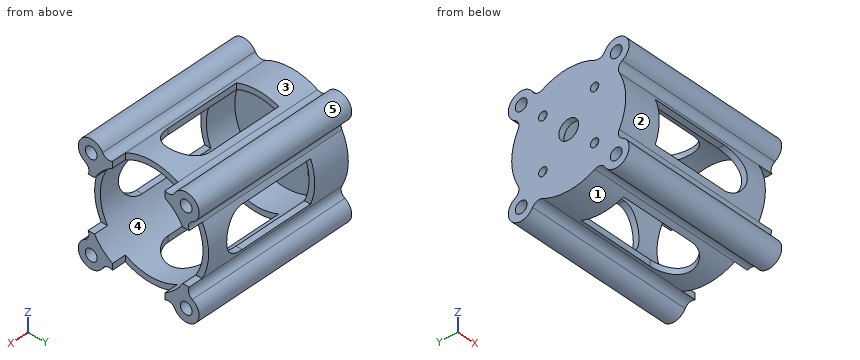
from build123d import *

# Parameters (mm, degrees)
SKETCH_1_R               = 20.25
EXTRUDE_1_DEPTH          = 2
SKETCH_2_R               = 3.5
CUT_EXTRUDE_1_DEPTH      = 3
SKETCH_3_R               = 20.25
SKETCH_3_R_2             = 10.25
EXTRUDE_2_DEPTH          = 4.1
SKETCH_5_R               = 20.25
SKETCH_5_R_2             = 16.25
EXTRUDE_3_DEPTH          = 5.4
SKETCH_6_R               = 20.25
SKETCH_6_R_2             = 18.25
EXTRUDE_4_DEPTH          = 47.5
SKETCH_7_R               = 1.5
CUT_EXTRUDE_2_DEPTH      = 60
PATTERN_CIRCULAR_1_COUNT = 4
FILLET_1_R               = 0.5
SKETCH_9_R               = 4.6
SKETCH_9_R_2             = 2.1
EXTRUDE_6_DEPTH          = 59
EXTRUDE_7_DEPTH          = 59
PATTERN_CIRCULAR_3_COUNT = 4
CUT_EXTRUDE_3_DEPTH      = 22.464496731
PATTERN_CIRCULAR_4_COUNT = 2
PATTERN_CIRCULAR_4_ANGLE = 270
SKETCH_22_R              = 18.25
CUT_EXTRUDE_9_DEPTH      = 20
SKETCH_23_W              = 5
SKETCH_23_H              = 18.640041254
CUT_EXTRUDE_10_DEPTH     = 43.928993463
PATTERN_CIRCULAR_5_COUNT = 2
PATTERN_CIRCULAR_5_ANGLE = 270


with BuildPart() as part:
    # Эскиз1 → Бобышка-Вытянуть1 (new body)
    with BuildSketch(Plane(origin=(0, 0, 0), x_dir=(0, 0, -1), z_dir=(1, 0, 0))):
        Circle(SKETCH_1_R)
    extrude(amount=EXTRUDE_1_DEPTH)

    # Эскиз2 → Вырез-Вытянуть1 (cut, through all)
    with BuildSketch(Plane.ZY):
        Circle(SKETCH_2_R)
    extrude(amount=-CUT_EXTRUDE_1_DEPTH, mode=Mode.SUBTRACT)

    # Эскиз3 → Бобышка-Вытянуть2 (add)
    with BuildSketch(Plane(origin=(2, 0, 0), x_dir=(0, 0, -1), z_dir=(1, 0, 0))):
        Circle(SKETCH_3_R)
        Circle(SKETCH_3_R_2, mode=Mode.SUBTRACT)
    extrude(amount=EXTRUDE_2_DEPTH)

    # Эскиз5 → Бобышка-Вытянуть3 (add)
    with BuildSketch(Plane(origin=(6.1, 0, 0), x_dir=(0, 0, -1), z_dir=(1, 0, 0))):
        Circle(SKETCH_5_R)
        Circle(SKETCH_5_R_2, mode=Mode.SUBTRACT)
    extrude(amount=EXTRUDE_3_DEPTH)

    # Эскиз6 → Бобышка-Вытянуть4 (add)
    with BuildSketch(Plane(origin=(11.5, 0, 0), x_dir=(0, 0, -1), z_dir=(1, 0, 0))):
        Circle(SKETCH_6_R)
        Circle(SKETCH_6_R_2, mode=Mode.SUBTRACT)
    extrude(amount=EXTRUDE_4_DEPTH)

    # Эскиз7 → Вырез-Вытянуть2 (cut, through all)
    with BuildSketch(Plane.ZY):
        with Locations((-9.192388155, 9.192388155)):
            Circle(SKETCH_7_R)
    cut_extrude_2 = extrude(amount=-CUT_EXTRUDE_2_DEPTH, mode=Mode.SUBTRACT)

    # Круговой массив1: Вырез-Вытянуть2 ×4 about axis
    pattern_circular_1_axis = Axis((0, 0, 0), (1, 0, 0))
    for i in range(1, PATTERN_CIRCULAR_1_COUNT):
        add(cut_extrude_2.rotate(pattern_circular_1_axis, i * 360 / PATTERN_CIRCULAR_1_COUNT), mode=Mode.SUBTRACT)

    # Скругление1
    fillet_1_edges = [part.edges().sort_by_distance(p)[0] for p in [
        (2, 0, 10.25),
        (6.1, 0, 10.25),
        (6.1, 0, 16.25),
        (11.5, 0, 16.25),
        (11.5, 0, 18.25),
    ]]
    fillet(fillet_1_edges, radius=FILLET_1_R)

    # Эскиз9 → Бобышка-Вытянуть6 (add)
    with BuildSketch(Plane.ZY):
        with Locations((-16.864496731, 16.864496731)):
            Circle(SKETCH_9_R)
        with Locations((-16.864496731, 16.864496731)):
            Circle(SKETCH_9_R_2, mode=Mode.SUBTRACT)
    extrude_6 = extrude(amount=-EXTRUDE_6_DEPTH)

    # Эскиз10 → Бобышка-Вытянуть7 (add)
    with BuildSketch(Plane.ZY):
        with BuildLine():
            ThreePointArc((-9.320020627, 17.977756131), (-11.289373131, 17.800047957), (-12.818708454, 19.053468456))
            ThreePointArc((-12.818708454, 19.053468456), (-12.323239372, 17.597287013), (-12.335539952, 16.059170405))
            ThreePointArc((-12.335539952, 16.059170405), (-10.870191755, 17.085123096), (-9.320020627, 17.977756131))
        make_face()
        with BuildLine():
            ThreePointArc((-16.059170405, 12.335539952), (-17.597287013, 12.323239372), (-19.053468456, 12.818708454))
            ThreePointArc((-19.053468456, 12.818708454), (-17.800047957, 11.289373131), (-17.977756131, 9.320020627))
            ThreePointArc((-17.977756131, 9.320020627), (-17.085123096, 10.870191755), (-16.059170405, 12.335539952))
        make_face()
    extrude_7 = extrude(amount=-EXTRUDE_7_DEPTH)

    # Круговой массив3: Бобышка-Вытянуть6, Бобышка-Вытянуть7 ×4 about axis
    pattern_circular_3_axis = Axis((0, 0, 0), (1, 0, 0))
    for i in range(1, PATTERN_CIRCULAR_3_COUNT):
        add(extrude_6.rotate(pattern_circular_3_axis, i * 360 / PATTERN_CIRCULAR_3_COUNT))
        add(extrude_7.rotate(pattern_circular_3_axis, i * 360 / PATTERN_CIRCULAR_3_COUNT))

    # Эскиз11 → Вырез-Вытянуть3 (cut, symmetric)
    with BuildSketch(Plane(origin=(0, 0, 0), x_dir=(1, 0, 0), z_dir=(0, 1, 0))):
        with BuildLine():
            Line((13, 7.5), (39.5, 7.5))
            ThreePointArc((39.5, 7.5), (47, 0), (39.5, -7.5))
            Line((39.5, -7.5), (13, -7.5))
            Line((13, -7.5), (13, 7.5))
        make_face()
    cut_extrude_3 = extrude(amount=CUT_EXTRUDE_3_DEPTH, both=True, mode=Mode.SUBTRACT)

    # Круговой массив4: Вырез-Вытянуть3 ×2 about axis
    pattern_circular_4_axis = Axis((2, 0, 0), (-1, 0, 0))
    for i in range(1, PATTERN_CIRCULAR_4_COUNT):
        add(cut_extrude_3.rotate(pattern_circular_4_axis, i * PATTERN_CIRCULAR_4_ANGLE / (PATTERN_CIRCULAR_4_COUNT - 1)), mode=Mode.SUBTRACT)

    # Эскиз22 → Вырез-Вытянуть9 (cut)
    with BuildSketch(Plane(origin=(2, 0, 0), x_dir=(0, 0, -1), z_dir=(1, 0, 0))):
        Circle(SKETCH_22_R)
    extrude(amount=CUT_EXTRUDE_9_DEPTH, mode=Mode.SUBTRACT)

    # Эскиз23 → Вырез-Вытянуть10 (cut, through all)
    with BuildSketch(Plane(origin=(0, -21.464496731, 0), x_dir=(-1, 0, 0), z_dir=(0, -1, 0))):
        with Locations((-56.5, 0)):
            Rectangle(SKETCH_23_W, SKETCH_23_H)
    cut_extrude_10 = extrude(amount=-CUT_EXTRUDE_10_DEPTH, mode=Mode.SUBTRACT)

    # Круговой массив5: Вырез-Вытянуть10 ×2 about axis
    pattern_circular_5_axis = Axis((2, 0, 0), (-1, 0, 0))
    for i in range(1, PATTERN_CIRCULAR_5_COUNT):
        add(cut_extrude_10.rotate(pattern_circular_5_axis, i * PATTERN_CIRCULAR_5_ANGLE / (PATTERN_CIRCULAR_5_COUNT - 1)), mode=Mode.SUBTRACT)


solid = part.part
Input: part model. Units: mm. Frame: model coordinates. Face numbers are marked on the shaded views. A direction names the side the tool comes from. Coordinates: 2 decimals unless noted, no trailing zeros. Loops run counter-clockwise (first coordinate to the right, second up) from the corner with the lowest first, then second, coordinate; pieces in that order, holes last.
(1) Section D-D on x = 10.5. Return the cut outline in (y, z), then the cut area to 3 significant figures.
(2) Section B-B on z = 5.5. Return the cut outline in (x, y), then the cut area to 3 significant figures.
(3) Pull-direction query (Z, two-part tool) for the marked faces 1, 2 and 3; classes: released by +Z, released by -Z, zero draft, split by the parting line, or undercut.
(4) Set-up query: the marked faces 4 and 5. Return all of +Z, -Z, +X, -X, +Y, -Y with unobstructed straight access to the full face (end or side cutting, diameter ignored); none if empty.
(5) Material intervals for probe 1 along Z at (x, y) = (39.5, -18); probe 2 along Y at (x, z) = (19.5, 15); probe 3 along X at (y, z) = (-5, -3), sorted ascending.
(6) Section A-A on y = 0. Return the cut outline in (x, z), then the cut area to 3 significant figures.
(7) First-contact query: pin 1 Ø1.4 at (y, z) = (-1, -18) entering from +X; pin 2 Ø3 at (x, z) = (51.5, 10) entering from -Y; pin 3 Ø1.1 at (x, y) = (22.5, 18) entering from -Z. Flat tips, straight axial feed; report the tip coordinate or a pass-through.
Data:
1. outline: (-19.05, -12.82) arc R4.6 ccw (long way) to (-12.82, -19.05) arc R2.61 cw to (-9.32, -17.98) arc R20.25 ccw to (9.32, -17.98) arc R2.61 cw to (12.82, -19.05) arc R4.6 ccw (long way) to (19.05, -12.82) arc R2.61 cw to (17.98, -9.32) arc R20.25 ccw to (17.98, 9.32) arc R2.61 cw to (19.05, 12.82) arc R4.6 ccw (long way) to (12.82, 19.05) arc R2.61 cw to (9.32, 17.98) arc R20.25 ccw to (-9.32, 17.98) arc R2.61 cw to (-12.82, 19.05) arc R4.6 ccw (long way) to (-19.05, 12.82) arc R2.61 cw to (-17.98, 9.32) arc R20.25 ccw to (-17.98, -9.32) arc R2.61 cw to start; hole circle Ø4.2 at (-16.86, -16.86); hole circle Ø4.2 at (-16.86, 16.86); hole circle Ø36.5 at (0, 0); hole circle Ø4.2 at (16.86, -16.86); hole circle Ø4.2 at (16.86, 16.86)
1. area: 457 mm2
2. outline: (0, -19.49) - (13, -19.49) - (13, -17.4) - (2, -17.4) - (2, 17.4) - (13, 17.4) - (13, 19.49) - (0, 19.49) - close; (44.6, -19.49) - (54, -19.49) - (54, -17.4) - (44.6, -17.4) - close; (44.6, 17.4) - (54, 17.4) - (54, 19.49) - (44.6, 19.49) - close
2. area: 163 mm2
3. face 1: released by -Z
3. face 2: undercut
3. face 3: released by +Z
4. face 4: +X
4. face 5: +X, -X
5. probe 1: z = -21.32 to -18.63, -15.1 to -11.77, -9.28 to -7.5, 7.5 to 9.28, 11.77 to 15.1, 18.63 to 21.32
5. probe 2: y = -21.07 to -17.83, -15.9 to -10.4, 10.4 to 15.9, 17.83 to 21.07
5. probe 3: x = 0 to 2
6. outline: (0, -20.25) - (13, -20.25) - (13, -18.25) - (2, -18.25) - (2, -3.5) - (0, -3.5) - close; (0, 3.5) - (2, 3.5) - (2, 18.25) - (13, 18.25) - (13, 20.25) - (0, 20.25) - close; (47, -20.25) - (54, -20.25) - (54, -18.25) - (47, -18.25) - close; (47, 18.25) - (54, 18.25) - (54, 20.25) - (47, 20.25) - close
6. area: 139 mm2
7. pin 1: stops at x = 54
7. pin 2: stops at y = -18.38
7. pin 3: stops at z = -21.43
